from build123d import *

# Parameters (mm, degrees)
SKETCH_1_W      = 14
SKETCH_1_H      = 9
EXTRUDE_1_DEPTH = 9
SKETCH_2_W      = 15
SKETCH_2_H      = 11
EXTRUDE_2_DEPTH = 1.5
SKETCH_3_W      = 11
SKETCH_3_H      = 7
EXTRUDE_3_DEPTH = 1.5
SKETCH_4_W      = 0.5
SKETCH_4_H      = 4
EXTRUDE_4_DEPTH = 8
FILLET_1_R      = 1
FILLET_2_R      = 0.5
FILLET_3_R      = 0.5
FILLET_4_R      = 0.5


with BuildPart() as part:
    # Эскиз1 → Бобышка-Вытянуть1 (new body)
    with BuildSketch(Plane(origin=(0, 0, 0), x_dir=(1, 0, 0), z_dir=(0, 1, 0))):
        Rectangle(SKETCH_1_W, SKETCH_1_H)
    extrude(amount=EXTRUDE_1_DEPTH)

    # Эскиз2 → Бобышка-Вытянуть2 (add)
    with BuildSketch(Plane(origin=(0, 9, 0), x_dir=(1, 0, 0), z_dir=(0, 1, 0))):
        Rectangle(SKETCH_2_W, SKETCH_2_H)
    extrude(amount=EXTRUDE_2_DEPTH)

    # Эскиз3 → Бобышка-Вытянуть3 (add)
    with BuildSketch(Plane(origin=(0, 10.5, 0), x_dir=(1, 0, 0), z_dir=(0, 1, 0))):
        Rectangle(SKETCH_3_W, SKETCH_3_H)
    extrude(amount=EXTRUDE_3_DEPTH)

    # Эскиз4 → Бобышка-Вытянуть4 (add)
    with BuildSketch(Plane.XZ):
        Rectangle(SKETCH_4_W, SKETCH_4_H)
        with Locations((5, 0)):
            Rectangle(SKETCH_4_W, SKETCH_4_H)
        with Locations((-5, 0)):
            Rectangle(SKETCH_4_W, SKETCH_4_H)
    extrude(amount=EXTRUDE_4_DEPTH)

    # Скругление1
    fillet_1_edges = [part.edges().sort_by_distance(p)[0] for p in [
        (7.5, 10.5, 0),
        (0, 10.5, -5.5),
        (-7.5, 10.5, 0),
        (0, 10.5, 5.5),
    ]]
    fillet(fillet_1_edges, radius=FILLET_1_R)

    # Скругление2
    fillet_2_edges = [part.edges().sort_by_distance(p)[0] for p in [
        (5.5, 12, 0),
        (0, 12, -3.5),
        (-5.5, 12, 0),
        (0, 12, 3.5),
    ]]
    fillet(fillet_2_edges, radius=FILLET_2_R)

    # Скругление3
    fillet_3_edges = [part.edges().sort_by_distance(p)[0] for p in [
        (0, 0, 4.5),
        (-7, 0, 0),
        (0, 0, -4.5),
        (7, 0, 0),
    ]]
    fillet(fillet_3_edges, radius=FILLET_3_R)

    # Скругление4
    fillet_4_edges = [part.edges().sort_by_distance(p)[0] for p in [
        (0, 0, -2),
        (0.25, 0, 0),
        (0, -8, 2),
        (0, -8, -2),
        (-0.25, 0, 0),
        (0, 0, 2),
        (5, 0, -2),
        (5.25, 0, 0),
        (5, -8, 2),
        (5, -8, -2),
        (4.75, 0, 0),
        (5, 0, 2),
        (-5, 0, -2),
        (-4.75, 0, 0),
        (-5, -8, 2),
        (-5, -8, -2),
        (-5.25, 0, 0),
        (-5, 0, 2),
    ]]
    fillet(fillet_4_edges, radius=FILLET_4_R)


solid = part.part
Design review of the part built by this model. Coordinates are the model's own, in mm. A direction names the side the tool comes from. Coordinates: 2 decimals unless noted, no trailing zeros. Write each loop counter-clockwise with the first axis right and the second up, starting at its lowest first coordinate (ties: lowest second). Pieces come first, ordered by that corner, then holes. Notation, with made-up numbers: (43, 88.5) - (61, 88.5) arc R30 cw to (61, 120.5) - close; hole circle Ø2 at (-32.75, 70.25). An arc over 180 degrees is marked (long way). One line per item, written item: value.
1) To check wall thickness, follow probe 1 along X at (y, z) = (-3.5, 1.5); probe 2 along Y at (x, z) = (-6.5, 3.75); probe 3 along X at (y, z) = (1.25, -0.75). State the ranges of each line that lie inside material, in increasing order.
Answer sheet:
probe 1: x = -5.25 to -4.75, -0.25 to 0.25, 4.75 to 5.25
probe 2: y = 0 to 10.5
probe 3: x = -7 to 7
2) Add section D-D (y = 2). State the section outline as (x, z) points.
Answer sheet:
outline: (-7, -4.5) - (7, -4.5) - (7, 4.5) - (-7, 4.5) - close
3) Mouldability with a two-part tool opening along X and no side actions: class faces 1 (the face through (0.25, -4, 0)), 2 (the face through (5.25, -4, 0)), 3 (the face through (0, 11, 3.5)), 4 (the face through (-0.25, -4, 0)) as +X half, -X half, draft (parallel to the pull), parting line (faces both ways), or undercut.
Answer sheet:
face 1: undercut
face 2: +X half
face 3: draft
face 4: undercut
4) Add section A-A (y = -2.75). State the section outline as (x, z) points.
Answer sheet:
outline: (-5.25, -2) - (-4.75, -2) - (-4.75, 2) - (-5.25, 2) - close; (-0.25, -2) - (0.25, -2) - (0.25, 2) - (-0.25, 2) - close; (4.75, -2) - (5.25, -2) - (5.25, 2) - (4.75, 2) - close
5) Add section B-B (x = 1). State the section outline as (y, z) points, plus the area to 3 significant figures.
Answer sheet:
outline: (0, -4) arc R0.5 ccw to (0.5, -4.5) - (9, -4.5) - (9, -5.5) - (9.5, -5.5) arc R1 ccw to (10.5, -4.5) - (10.5, -3.5) - (11.5, -3.5) arc R0.5 ccw to (12, -3) - (12, 3) arc R0.5 ccw to (11.5, 3.5) - (10.5, 3.5) - (10.5, 4.5) arc R1 ccw to (9.5, 5.5) - (9, 5.5) - (9, 4.5) - (0.5, 4.5) arc R0.5 ccw to (0, 4) - close
area: 107 mm2
6) For faces 5 (the face through (7, 5, 0)), 6 (the face through (4.75, -4, 0)), 7 (the face through (-7, 5, 0)), list the 3-axis set-ups (+Z, -Z, +X, -X, +Y, -Y) from which the entire face can be reached by the end or side of a thin tool; tool diameter is ignored.
Answer sheet:
face 5: +Z, -Z, +X, -Y
face 6: +Z, -Z, -Y
face 7: +Z, -Z, -X, -Y
7) Add section C-C (z = -4.25). State the section outline as (x, y) points.
Answer sheet:
outline: (-7.5, 9) - (-7, 9) - (-7, 0.5) arc R0.5 ccw to (-6.75, 0.07) - (6.75, 0.07) arc R0.5 ccw to (7, 0.5) - (7, 9) - (7.5, 9) - (7.5, 9.5) arc R1 ccw to (6.5, 10.5) - (-6.5, 10.5) arc R1 ccw to (-7.5, 9.5) - close
8) Insertion check: pin 1 (1.2 mm diameter, centred on y = -6, z = 0.5, fed in from +X); pin 2 (3 mm diameter, centred on x = -1, y = -1, fed in from -Z); pin 3 (6 mm diameter, centred on y = 2, z = 2, fed in from -X). Each pin has a flat end and moves straight along its axis. Give the tip position at first contact, or say it passes through.
Answer sheet:
pin 1: stops at x = 5.25
pin 2: stops at z = -4.5
pin 3: stops at x = -7
